Verification items for the finished model (mm, model axes). Coordinates: 2 decimals unless noted, no trailing zeros. Order: outer loops, then holes, each group sorted by start corner. A loop starts at its lowest first (then second) coordinate and runs counter-clockwise, first axis right, second up. Notation, with made-up numbers: M -36.75,9 L -7.75,9 A23 ccw -7.75,41 Z; hole C -7.75,46 d6. An arc over 180 degrees is marked long. Return JSON: item names as keys, results as strings. Group by question number.
Q1. Mould release check, pull along X, two halves, no side actions. Record for faces 1 (the face through (-0.066, 6.405, -1.632)), 2 (the face through (-1, 8, 1.588)), 3 (the face through (1.86, 6, 3)): pulls with the +X half, pulls with the -X half, needs draft (parallel to the pull), parting line crosses it, or undercut.
Q2. Section check A-A, the plane x = -0.5. Enter the section's corners in (y, z).
Q3. Thickness scan on probe 1 along Y at (x, z) = (-0.75, -3.25); probe 2 along X at (y, z) = (6.35, -1.5); probe 3 along X at (y, z) = (6, -1.5). Record the ranges inside material, lowest first.
Q4. Go/stop test with flat-tipped pins: pin 1 Ø5 at (x, y) = (-1, 8.5) entering from +Z; pin 2 Ø2 at (y, z) = (10, 2.5) entering from -X; pin 3 Ø3 at (y, z) = (8.5, 2.5) entering from -X. Record where each tip stops, or that it passes through.
Q5. Section check D-D, the plane y = 11. Enter the section's corners in (x, z) (1 decimal).
Q6. Section check C-C, the plane y = 6.35. Enter the section's corners in (x, z) (1 decimal).
Q7. Section check B-B, the plane z = 0. Enter the section's corners in (x, y), then the cut area to 3 significant figures.
from build123d import *

# Parameters (mm, degrees)
PROFILE_SKETCH_R       = 4.7625
BOSS_EXTRUDE1_DEPTH    = 12.7
PLATE_RELIEF_CUT_REACH = 14.7
PLATE_RELIEF_SKETCH_W  = 6.35
PLATE_RELIEF_SKETCH_H  = 3.175
M3X0_5_TAPPED_HOLE1_D  = 2.5


with BuildPart() as part:
    # Profile Sketch → Boss-Extrude1 (new body)
    with BuildSketch(Plane(origin=(0, 0, 0), x_dir=(1, 0, 0), z_dir=(0, 1, 0))):
        Circle(PROFILE_SKETCH_R)
    extrude(amount=BOSS_EXTRUDE1_DEPTH)

    # Plate Relief Sketch → Plate Relief Cut (cut, up to next)
    with BuildSketch(Plane.XZ, mode=Mode.PRIVATE) as plate_relief_cut_sk1:
        with Locations((-1.315128061, 3.175)):
            Rectangle(PLATE_RELIEF_SKETCH_W, PLATE_RELIEF_SKETCH_H)
    plate_relief_cut_tool1 = extrude(plate_relief_cut_sk1.sketch, amount=-PLATE_RELIEF_CUT_REACH, mode=Mode.PRIVATE) & part.part
    add(plate_relief_cut_tool1.solids().sort_by_distance((-1.315128, 0, 3.175))[0], mode=Mode.SUBTRACT)

    # M3x0.5 Tapped Hole1 (through all)
    with Locations(Plane(origin=(-1.315128061, 6.35, 1.5875), x_dir=(1, 0, 0), z_dir=(0, 0, 1))):
        with Locations((0, 0)):
            Hole(M3X0_5_TAPPED_HOLE1_D / 2)


solid = part.part
Numbers:
{
 "1": {"face 1": "undercut", "face 2": "needs draft", "face 3": "pulls with the -X half"},
 "2": {"outline": "M 0,-4.74 L 5.4,-4.74 L 5.4,1.59 L 0,1.59 Z; M 7.3,-4.74 L 12.7,-4.74 L 12.7,1.59 L 7.3,1.59 Z"},
 "3": {"probe 1": "y = 0 to 5.24, 7.46 to 12.7", "probe 2": "x = -4.52 to -2.57, -0.07 to 4.52", "probe 3": "x = -4.52 to -2.52, -0.12 to 4.52"},
 "4": {"pin 1": "stops at z = 1.59", "pin 2": "stops at x = -4.52", "pin 3": "stops at x = -4.66"},
 "5": {"outline": "M -4.5,1.6 A4.8 ccw long 1.9,4.4 L 1.9,1.6 Z"},
 "6": {"outline": "M -4.5,1.6 A4.8 ccw -2.6,-4 L -2.6,1.6 Z; M -0.1,-4.8 A4.8 ccw 1.9,4.4 L 1.9,1.6 L -0.1,1.6 Z"},
 "7": {"outline": "M -4.76,0 L 4.76,0 L 4.76,12.7 L -4.76,12.7 Z; hole C -1.32,6.35 d2.5", "area": "116 mm2"}
}
